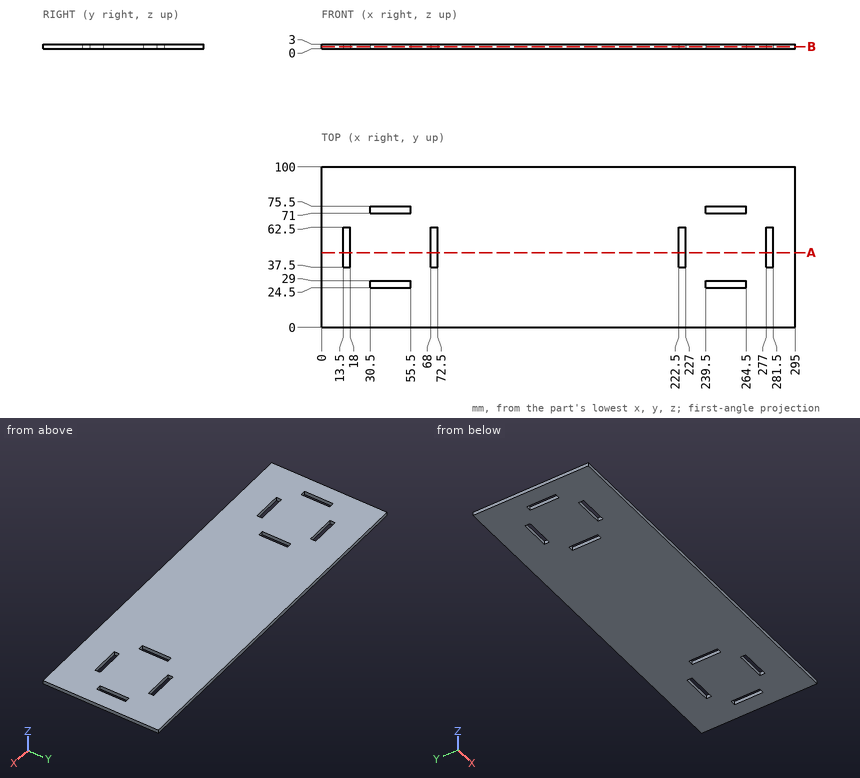
Verification items for this drawing (mm, ordinates from the low corner). Coordinates: 2 decimals unless noted, no trailing zeros. Write each loop counter-clockwise with the first axis right and the second up, starting at its lowest first coordinate (ties: lowest second). Pieces come first, ordered by that corner, then holes. Notation, with made-up numbers: M 75,19 L 110,19 A12 cw 110,37 Z; hole C -2.5,9 d6. An arc over 180 degrees is marked long. Answer as CSV lines item,"result".
Q1. Cross-section at B-B (z = 1.3). Count the separate pieces of the cut face and the enclosed holes in it, then the cut area to 3 significant figures.
Check result:
separate pieces,"1"
enclosed holes,"8"
area,"28,600 mm^2"
Q2. Go/stop test with a flat-tipped pin: pin 1 (6 mm diameter, centred on x = 169.5, y = 13.5, fed in from -Z). Record where the tip stops, or that it passes through.
Check result:
pin 1,"z = 0"
Q3. Cross-section at A-A (y = 46.5). Record the boundary of the cut face in (x, z).
Check result:
outline,"M 0,0 L 13.5,0 L 13.5,3 L 0,3 Z; M 18,0 L 68,0 L 68,3 L 18,3 Z; M 72.5,0 L 222.5,0 L 222.5,3 L 72.5,3 Z; M 227,0 L 277,0 L 277,3 L 227,3 Z; M 281.5,0 L 295,0 L 295,3 L 281.5,3 Z"
Q4. Material ranges on probe 1 along X at (y, z) = (56, 0.2); probe 2 along X at (y, z) = (28, 1.65); probe 3 along Y at (x, z) = (255, 2.45), recorded low to high. Write a range as from..to.
Check result:
probe 1,"0..13.5, 18..68, 72.5..222.5, 227..277, 281.5..295"
probe 2,"0..30.5, 55.5..239.5, 264.5..295"
probe 3,"0..24.5, 29..71, 75.5..100"
